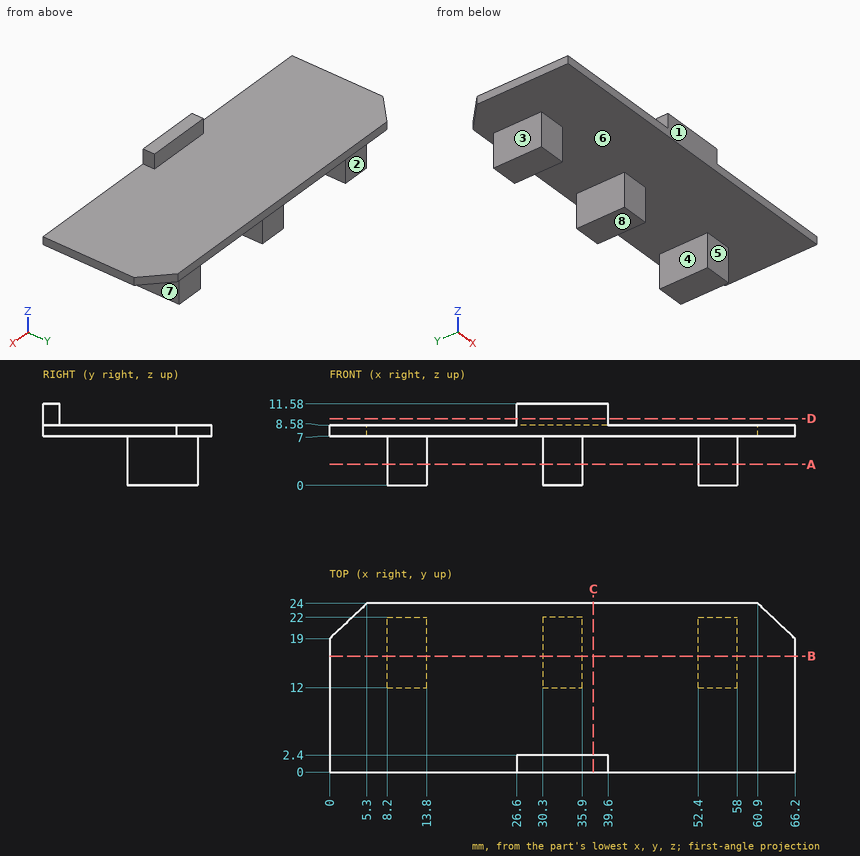
Print and shaded views of the part. All mm, measured from the part's lowest x, y and z. A direction names the side the tool comes from. Coordinates: 2 decimals unless noted, no trailing zeros. Write each loop counter-clockwise with the first axis right and the second up, starting at its lowest first coordinate (ties: lowest second). Pieces come first, ordered by that corner, then holes.
(1) 3-axis set-ups, long thin cutter, end or side, ignore diameter. For the marked faces 1, 2, 3, 4 and 5: which of +Z, -Z, +X, -X, +Y, -Y reach the whole face in a straight line?
(2) Cut at A-A, the plane z = 3. List the corners of the cut face in (x, y).
(3) Drill centre lines: probe 1 along X at (y, z) = (14, 2.25); probe 2 along Z at (x, y) = (21.5, 22.5); probe 3 along Y at (x, z) = (13, 3). Where is each one in solid material? Low to high.
(4) Flat gauge pins, fed straight in: pin 1 (4.5 mm diameter, centred on x = 32, z = 4, fed in from -Y); pin 2 (3 mm diameter, centred on x = 34.5, z = 4.5, fed in from +Y); pin 3 (5.5 mm diameter, centred on y = 15.5, z = 2.5, fed in from -X). Where does each tip first touch, or does it go through?
(5) Two-plate mould, pull along X, no slides. Class the marked faces 6, 7 and 8: +X half, -X half, draft (parallel to the pull), parting line (faces both ways), or undercut.
(6) Cut at C-C, the plane x = 37.5. List the corners of the cut face in (y, z), and give its area (3 significant figures).
(7) Cut at D-D, the plane z = 9.5. List the corners of the cut face in (x, y), and give its area (3 significant figures).
(8) Cut at B-B, the plane y = 16.5. List the corners of the cut face in (x, z), and give its area (3 significant figures).
Geometry says:
1. face 1: +Z, -Z, +X, -X, -Y
1. face 2: -Z, +X, -X, +Y
1. face 3: -Z, -X, +Y, -Y
1. face 4: -Z, +Y, -Y
1. face 5: -Z, +X, -X, -Y
2. outline: (8.2, 12) - (13.8, 12) - (13.8, 22) - (8.2, 22) - close; (30.3, 12) - (35.9, 12) - (35.9, 22) - (30.3, 22) - close; (52.4, 12) - (58, 12) - (58, 22) - (52.4, 22) - close
3. probe 1: x = 8.2 to 13.8, 30.3 to 35.9, 52.4 to 58
3. probe 2: z = 7 to 8.58
3. probe 3: y = 12 to 22
4. pin 1: stops at y = 12
4. pin 2: stops at y = 22
4. pin 3: stops at x = 8.2
5. face 6: undercut
5. face 7: +X half
5. face 8: draft
6. outline: (0, 7) - (24, 7) - (24, 8.58) - (2.4, 8.58) - (2.4, 11.58) - (0, 11.58) - close
6. area: 45.1 mm2
7. outline: (26.6, 0) - (39.6, 0) - (39.6, 2.4) - (26.6, 2.4) - close
7. area: 31.2 mm2
8. outline: (0, 7) - (8.2, 7) - (8.2, 0) - (13.8, 0) - (13.8, 7) - (30.3, 7) - (30.3, 0) - (35.9, 0) - (35.9, 7) - (52.4, 7) - (52.4, 0) - (58, 0) - (58, 7) - (66.2, 7) - (66.2, 8.58) - (0, 8.58) - close
8. area: 222 mm2
